from build123d import *

# Parameters (mm, degrees)
BOSS_EXTRUDE1_DEPTH = 70
SKETCH2_R           = 3.2639
CUT_EXTRUDE1_DEPTH  = 70
SKETCH3_R           = 17.5
CUT_EXTRUDE2_DEPTH  = 71


with BuildPart() as part:
    # Sketch1 → Boss-Extrude1 (new body)
    with BuildSketch(Plane(origin=(0, 0, 0), x_dir=(1, 0, 0), z_dir=(0, 1, 0))):
        with BuildLine():
            Line((0, -5), (0, -85))
            Line((0, -85), (5, -85))
            Line((5, -85), (5, 0))
            ThreePointArc((5, 0), (3.535533906, 3.535533906), (0, 5))
            Line((0, 5), (-1, 5))
            ThreePointArc((-1, 5), (-4.535533906, 6.464466094), (-6, 10))
            Line((-6, 10), (-6, 47.65))
            Line((-6, 47.65), (-11, 47.65))
            Line((-11, 47.65), (-11, 5))
            ThreePointArc((-11, 5), (-9.535533906, 1.464466094), (-6, 0))
            Line((-6, 0), (-5, 0))
            ThreePointArc((-5, 0), (-1.464466094, -1.464466094), (0, -5))
        make_face()
    extrude(amount=BOSS_EXTRUDE1_DEPTH)

    # Sketch2 → Cut-Extrude1 (cut)
    with BuildSketch(Plane(origin=(-6, 0, 0), x_dir=(0, 0, -1), z_dir=(1, 0, 0))):
        with Locations((37.65, 58.8125)):
            Circle(SKETCH2_R)
        with Locations((37.65, 11.1875)):
            Circle(SKETCH2_R)
    extrude(amount=-CUT_EXTRUDE1_DEPTH, mode=Mode.SUBTRACT)

    # Sketch3 → Cut-Extrude2 (cut, through all)
    with BuildSketch(Plane(origin=(0, 70, 0), x_dir=(1, 0, 0), z_dir=(0, 1, 0))):
        with Locations((2.5, -79)):
            Circle(SKETCH3_R)
    extrude(amount=-CUT_EXTRUDE2_DEPTH, mode=Mode.SUBTRACT)


solid = part.part
Source: CAD feature listing. Evaluate the final solid. Frame: model axes, mm. A direction names the side the tool comes from. Coordinates: 2 decimals unless noted, no trailing zeros. Loops run counter-clockwise (first coordinate to the right, second up) from the corner with the lowest first, then second, coordinate; pieces in that order, holes last. Notation, with made-up numbers: (79, 8) - (134, 8) arc R24 cw to (134, 31) - close; hole circle Ø5 at (-23.75, 8.25). An arc over 180 degrees is marked (long way). One line per item, written item: value. Start each with the question number.
1. Ray query, L1, parallel to Y at x = -7.55, z = -37.65; L2, parallel to X at y = 50, z = 19.5; L3, parallel to X at y = 65.5, z = -31. Return the intervals inside material, ascending.
2. Section B-B (y = 5). Return the cut outline in (x, z), and give its area (3 significant figures).
3. Mould query, pull axis Y, two halves, no side actions, for faces 4 (the flat face through (0, 0, 3)), 5 (the cylindrical face through (-8.465, 55.626, -36.942)), 6 (the cylindrical face through (-2, 35, 1)). Classes: pulls with the +Y half, pulls with the -Y half, needs draft (parallel to the pull), parting line crosses it, or undercut.
4. Section A-A (z = -37.65). Return the cut outline in (x, y).
5. Set-up query: faces 1 (the flat face through (-6, 35, -29)), 2 (the cylindrical face through (-8.46, 11.33, -34.39)), 3 (the flat face through (0, 35, 33)). Return all of +Z, -Z, +X, -X, +Y, -Y with unobstructed straight access to the full face (end or side cutting, diameter ignored); none if empty.
6. Section D-D (x = 1.5). Return the cut outline in (y, z), and give its area (3 significant figures).
7. Contact query for flat-ended pins moving along their axis: P1, Ø6, axis at y = 61, z = -28, coming from the +X side; P2, Ø5, axis at y = 58.81, z = -37.65, coming from the +X side; P3, Ø2, axis at y = 34, z = 22, coming from the -X side. Output: stop coordinate, or through.
8. Section C-C (z = 27). Return the cut outline in (x, y).
Verdict:
1. L1: y = 0 to 7.92, 14.45 to 55.55, 62.08 to 70
1. L2: x = 0 to 5
1. L3: x = -11 to -6
2. outline: (-11, -47.65) - (-6, -47.65) - (-6, -10) arc R5 cw to (-1, -5) - (0, -5) arc R5 ccw to (5, 0) - (5, 61.68) arc R17.5 cw to (0, 61.68) - (0, 5) arc R5 cw to (-5, 0) - (-6, 0) arc R5 ccw to (-11, -5) - close
2. area: 601 mm2
3. face 4: pulls with the -Y half
3. face 5: undercut
3. face 6: needs draft
4. outline: (-11, 0) - (-6, 0) - (-6, 7.92) - (-11, 7.92) - close; (-11, 14.45) - (-6, 14.45) - (-6, 55.55) - (-11, 55.55) - close; (-11, 62.08) - (-6, 62.08) - (-6, 70) - (-11, 70) - close
5. face 1: -Z, +X, +Y, -Y
5. face 2: +X, -X
5. face 3: +Z, -X, +Y, -Y
6. outline: (0, -4.77) - (70, -4.77) - (70, 61.53) - (0, 61.53) - close
6. area: 4,640 mm2
7. P1: stops at x = -6
7. P2: passes through
7. P3: stops at x = 0
8. outline: (0, 0) - (5, 0) - (5, 70) - (0, 70) - close
